Verification items for the finished model (mm, model axes). Coordinates: 2 decimals unless noted, no trailing zeros. Order: outer loops, then holes, each group sorted by start corner. A loop starts at its lowest first (then second) coordinate and runs counter-clockwise, first axis right, second up. Notation, with made-up numbers: (7.25, -22) -> (45.25, -22) arc R23 cw to (45.25, 11) -> close; hole circle Ø8 at (-25, 41). An arc over 180 degrees is marked (long way). Write item = value, one per line. Start each with the question number.
1. Go/stop test with flat-tipped pins: P1, Ø3, axis at x = 1.5, z = 2.5, coming from the +Y side; P2, Ø3, axis at y = 43, z = 3, coming from the +X side; P3, Ø1.5, axis at x = -11.5, z = 6, coming from the +Y side; P4, Ø5, axis at x = -2, y = 99, coming from the +Z side. Record where each tip stops, or that it passes through.
2. Cross-section at B-B on x = 0. Record the cut outline in (y, z).
3. Cross-section at D-D on x = -26. Record the cut outline in (y, z), plus the area to 3 significant figures.
4. Cross-section at C-C on y = 14. Record the cut outline in (x, z), plus the area to 3 significant figures.
5. Cross-section at A-A on z = 1.5. Record the cut outline in (x, y).
6. Thickness scan on line 1 along Y through (x, z) = (0, 3.8); line 2 along X through (y, z) = (16, 2.25); line 3 along X through (y, z) = (45.5, 2.75). Record the ranges inside material, lowest first. Write a range as from..to.
from build123d import *

# Parameters (mm, degrees)
SKETCH1_R           = 12.5
BOSS_EXTRUDE1_DEPTH = 6.5
CUT_EXTRUDE1_REACH  = 124.839
SKETCH2_R           = 3.5
SKETCH2_3_R         = 8
SKETCH2_3_R_2       = 3.5
CUT_EXTRUDE2_DEPTH  = 4
CUT_EXTRUDE4_REACH  = 124.839
SKETCH3_R           = 2


with BuildPart() as part:
    # Sketch1 → Boss-Extrude1 (new body)
    with BuildSketch(Plane.XY):
        with Locations((0, 100)):
            Circle(SKETCH1_R)
        with BuildLine():
            Line((-48.897023427, 0), (48.897023427, 0))
            Line((48.897023427, 0), (12.5, 100))
            ThreePointArc((12.5, 100), (10.716279715, 93.564834962), (5.87418415, 88.966235431))
            Line((5.87418415, 88.966235431), (34.615543359, 10))
            Line((34.615543359, 10), (-34.615543359, 10))
            Line((-34.615543359, 10), (-5.87418415, 88.966235431))
            ThreePointArc((-5.87418415, 88.966235431), (-10.716279715, 93.564834962), (-12.5, 100))
            Line((-12.5, 100), (-48.897023427, 0))
        make_face()
        with BuildLine():
            Line((-5, 10), (5, 10))
            Line((5, 10), (5, 88.543560763))
            ThreePointArc((5, 88.543560763), (0, 87.5), (-5, 88.543560763))
            Line((-5, 88.543560763), (-5, 10))
        make_face()
    extrude(amount=BOSS_EXTRUDE1_DEPTH)

    # Sketch2 → Cut-Extrude1 (cut, up to next)
    with BuildSketch(Plane.XY.offset(6.5), mode=Mode.PRIVATE) as cut_extrude1_sk1:
        with Locations((0, 100)):
            Circle(SKETCH2_R)
    cut_extrude1_tool1 = extrude(cut_extrude1_sk1.sketch, amount=-CUT_EXTRUDE1_REACH, mode=Mode.PRIVATE) & part.part
    add(cut_extrude1_tool1.solids().sort_by_distance((0, 100, 6.5))[0], mode=Mode.SUBTRACT)

    # Sketch2<3> → Cut-Extrude2 (cut)
    with BuildSketch(Plane.XY.offset(6.5)):
        with Locations((0, 100)):
            Circle(SKETCH2_3_R)
        with Locations((0, 100)):
            Circle(SKETCH2_3_R_2, mode=Mode.SUBTRACT)
    extrude(amount=-CUT_EXTRUDE2_DEPTH, mode=Mode.SUBTRACT)

    # Sketch3 → Cut-Extrude4 (cut, up to next)
    with BuildSketch(Plane.XY.offset(6.5), mode=Mode.PRIVATE) as cut_extrude4_sk1:
        with Locations((0, 5)):
            Circle(SKETCH3_R)
    cut_extrude4_tool1 = extrude(cut_extrude4_sk1.sketch, amount=-CUT_EXTRUDE4_REACH, mode=Mode.PRIVATE) & part.part
    # Sketch3 → Cut-Extrude4 (cut, up to next)
    with BuildSketch(Plane.XY.offset(6.5), mode=Mode.PRIVATE) as cut_extrude4_sk2:
        with Locations((40.397023427, 5)):
            Circle(SKETCH3_R)
    cut_extrude4_tool2 = extrude(cut_extrude4_sk2.sketch, amount=-CUT_EXTRUDE4_REACH, mode=Mode.PRIVATE) & part.part
    # Sketch3 → Cut-Extrude4 (cut, up to next)
    with BuildSketch(Plane.XY.offset(6.5), mode=Mode.PRIVATE) as cut_extrude4_sk3:
        with Locations((-40.397023427, 5)):
            Circle(SKETCH3_R)
    cut_extrude4_tool3 = extrude(cut_extrude4_sk3.sketch, amount=-CUT_EXTRUDE4_REACH, mode=Mode.PRIVATE) & part.part
    # Sketch3 → Cut-Extrude4 (cut, up to next)
    with BuildSketch(Plane.XY.offset(6.5), mode=Mode.PRIVATE) as cut_extrude4_sk4:
        with Locations((0, 25)):
            Circle(SKETCH3_R)
    cut_extrude4_tool4 = extrude(cut_extrude4_sk4.sketch, amount=-CUT_EXTRUDE4_REACH, mode=Mode.PRIVATE) & part.part
    add(cut_extrude4_tool1.solids().sort_by_distance((0, 5, 6.5))[0], mode=Mode.SUBTRACT)
    add(cut_extrude4_tool2.solids().sort_by_distance((40.397023, 5, 6.5))[0], mode=Mode.SUBTRACT)
    add(cut_extrude4_tool3.solids().sort_by_distance((-40.397023, 5, 6.5))[0], mode=Mode.SUBTRACT)
    add(cut_extrude4_tool4.solids().sort_by_distance((0, 25, 6.5))[0], mode=Mode.SUBTRACT)


solid = part.part
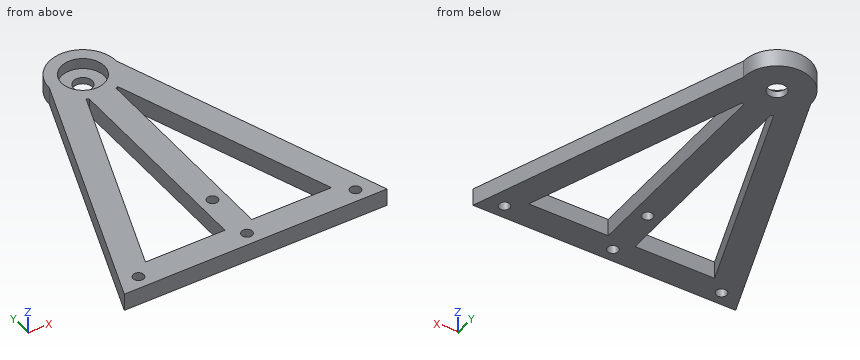
Worked out:
q1.P1 = 112.5
q1.P2 = 33.79
q1.P3 = 106.38
q1.P4 = 2.5
q2.outline = (0, 0) -> (3, 0) -> (3, 6.5) -> (0, 6.5) -> close; (7, 0) -> (23, 0) -> (23, 6.5) -> (7, 6.5) -> close; (27, 0) -> (96.5, 0) -> (96.5, 2.5) -> (92, 2.5) -> (92, 6.5) -> (27, 6.5) -> close; (103.5, 0) -> (112.5, 0) -> (112.5, 6.5) -> (108, 6.5) -> (108, 2.5) -> (103.5, 2.5) -> close
q3.outline = (0, 0) -> (10, 0) -> (10, 6.5) -> (0, 6.5) -> close; (33.67, 0) -> (62.91, 0) -> (62.91, 6.5) -> (33.67, 6.5) -> close
q3.area = 255 mm²
q4.outline = (-43.8, 0) -> (-33.16, 0) -> (-33.16, 6.5) -> (-43.8, 6.5) -> close; (-5, 0) -> (5, 0) -> (5, 6.5) -> (-5, 6.5) -> close; (33.16, 0) -> (43.8, 0) -> (43.8, 6.5) -> (33.16, 6.5) -> close
q4.area = 203 mm²
q5.outline = (-48.9, 0) -> (48.9, 0) -> (12.5, 100) arc R12.5 ccw to (-12.5, 100) -> close; hole circle Ø4 at (-40.4, 5); hole (-34.62, 10) -> (-5, 10) -> (-5, 88.54) arc R12.5 cw to (-5.87, 88.97) -> close; hole circle Ø7 at (0, 100); hole circle Ø4 at (0, 5); hole circle Ø4 at (0, 25); hole (5, 10) -> (34.62, 10) -> (5.87, 88.97) arc R12.5 cw to (5, 88.54) -> close; hole circle Ø4 at (40.4, 5)
q6.line_1 = 0..3, 7..23, 27..92, 108..112.5
q6.line_2 = -43.07..-32.43, -5..5, 32.43..43.07
q6.line_3 = -32.34..-21.69, -5..5, 21.69..32.34
